Autodesk Inventor part; units mm, degrees
ref_plane "YZ Plane" through (0, 0, 0) normal (1, 0, 0) x (0, 1, 0)
ref_plane "XZ Plane" through (0, 0, 0) normal (0, 1, 0) x (-1, 0, 0)
ref_plane "XY Plane" through (0, 0, 0) normal (0, 0, 1) x (1, 0, 0)
sketch "草图1" plane through (0, 0, 0) normal (0, 0, 1) x (1, 0, 0)
  arc A0 (25, -75) -> (-25, -75) centre (0, -75) ccw
  line L0 (-25, -75) -> (-25, -96.8246)
  line L1 (25, -75) -> (25, -96.8246)
  line L2 (0, 0) -> (9.4022, 0)
  line L3 (0, 0) -> (0, -9.3611)
  arc A1 (75, 25) -> (75, -25) centre (75, 0) ccw
  line L4 (75, -25) -> (96.8246, -25)
  line L5 (75, 25) -> (96.8246, 25)
  arc A2 (-25, 75) -> (25, 75) centre (0, 75) ccw
  line L6 (25, 75) -> (25, 96.8246)
  line L7 (-25, 75) -> (-25, 96.8246)
  arc A3 (-75, -25) -> (-75, 25) centre (-75, 0) ccw
  line L8 (-75, 25) -> (-96.8246, 25)
  line L9 (-75, -25) -> (-96.8246, -25)
  arc A4 (-25, 96.8246) -> (-96.8246, 25) centre (0, 0) ccw
  arc A5 (96.8246, 25) -> (25, 96.8246) centre (0, 0) ccw
  arc A6 (-96.8246, -25) -> (-25, -96.8246) centre (0, 0) ccw
  arc A7 (25, -96.8246) -> (96.8246, -25) centre (0, 0) ccw
  dimension "d0" = 50
  dimension "d2" = 9.4022
  dimension "d3" = 9.3611
  dimension "d6" = 360
  dimension "d12" = 100
extrude "拉伸1" add sketch "草图1" along normal blind 28
sketch "草图2" plane through (0, 0, 28) normal (0, 0, 1) x (1, 0, 0)
  circle A0 centre (0, 0) radius 25
  arc A1 (30, -75) -> (-30, -75) centre (0, -75) ccw
  arc A2 (25, -75) -> (-25, -75) centre (0, -75) ccw
  line L0 (30, -75) -> (30, -90.1388)
  line L1 (-30, -75) -> (-30, -90.1388)
  arc A3 (75, 30) -> (75, -30) centre (75, 0) ccw
  line L2 (75, 30) -> (90.1388, 30)
  line L3 (75, -30) -> (90.1388, -30)
  arc A4 (-30, 75) -> (30, 75) centre (0, 75) ccw
  line L4 (-30, 75) -> (-30, 90.1388)
  line L5 (30, 75) -> (30, 90.1388)
  arc A5 (-75, -30) -> (-75, 30) centre (-75, 0) ccw
  line L6 (-75, -30) -> (-90.1388, -30)
  line L7 (-75, 30) -> (-90.1388, 30)
  arc A6 (-90.1388, -30) -> (-30, -90.1388) centre (0, 0) ccw
  arc A7 (-30, 90.1388) -> (-90.1388, 30) centre (0, 0) ccw
  arc A8 (30, -90.1388) -> (90.1388, -30) centre (0, 0) ccw
  arc A9 (90.1388, 30) -> (30, 90.1388) centre (0, 0) ccw
  dimension "d15" = 50
  dimension "d17" = 5
  dimension "d20" = 360
  dimension "d22" = 95
extrude "拉伸2" cut sketch "草图2" against normal blind 9
pattern_linear "矩形阵列1" count 2 spacing 19 along (0, 0, -1) of "拉伸2"
sketch "草图3" plane through (0, 0, 28) normal (0, 0, 1) x (1, 0, 0)
  circle A0 centre (0, 0) radius 15
  line L0 (-4, 14.4568) -> (4, 14.4568)
  line L1 (4, 14.4568) -> (4, 17.2)
  line L2 (4, 17.2) -> (-4, 17.2)
  line L3 (-4, 17.2) -> (-4, 14.4568)
  dimension "d28" = 30
  dimension "d29" = 17.2
  dimension "d30" = 8
extrude "拉伸3" cut sketch "草图3" against normal blind 28
properties part number "基准图-装填桶"
Geometry: final body of the model. Coordinates: model frame, mm. A direction names the side the tool comes from. Round coordinates to 2 decimals unless told otherwise and drop trailing zeros. Loops run counter-clockwise (first coordinate to the right, second up) from the corner with the lowest first, then second, coordinate; pieces in that order, holes last. Notation, with made-up numbers: M 79,35 L 116,35 A18 cw 116,46 Z; hole C 53,10.25 d6. An arc over 180 degrees is marked long. Put each result on its own line as item: value. Start each with the question number.
(1) Section query A-A (y = 0). Return loops of the section in (x, z).
(2) Draft query along Y for faces 1 (the face through (70.18, 71.24, 13.8)), 2 (the face through (66.74, -67.61, 4.56)), 3 (the face through (-0.5, -49.8, 0)). Return one class per face: +Y half, -Y half, draft (parallel to the pull), parting line (faces both ways), or undercut.
(3) Section query D-D (x = 40.5). Return loops of the section in (y, z), then the cut area to 3 significant figures.
(4) Section query C-C (z = 2.5). State how many separate pieces and enclosed holes the cut face has, then the cut area to 3 significant figures.
(5) Set-up query: faces 4 (the face through (25, -86, 14)), 5 (the face through (25, 86, 14)), 6 (the face through (-86, 25, 14)), 7 (the face through (-82, -30, 24)), 8 (the face through (45.007, 0.66, 4.563)). Return all of +Z, -Z, +X, -X, +Y, -Y with unobstructed straight access to the full face (end or side cutting, diameter ignored); none if empty.
(6) Section query B-B (x = -70). Return loops of the section in (y, z), then the cut area to 3 significant figures.
(7) Contact query for flat-ended pins moving along their axis: pin 1 Ø7 at (x, z) = (82.5, 25.5) entering from +Y; pin 2 Ø7 at (x, z) = (-82.5, 22.5) entering from -Y; pin 3 Ø6.5 at (x, z) = (89, 9) entering from -Y. Output: stop coordinate, or through.
(8) Material intervals for line 1 along X through (y, z) = (0, 16.75); line 2 along X through (y, z) = (-85.5, 26.75); line 3 along Y through (x, z) = (-5.5, 2.5), sorted ascending. Write a range as [from, to].
Findings below:
1. outline: M -50,0 L -45,0 L -45,9 L -25,9 L -25,0 L -15,0 L -15,28 L -25,28 L -25,19 L -45,19 L -45,28 L -50,28 Z; M 15,0 L 25,0 L 25,9 L 45,9 L 45,0 L 50,0 L 50,28 L 45,28 L 45,19 L 25,19 L 25,28 L 15,28 Z
2. face 1: +Y half
2. face 2: undercut
2. face 3: draft
3. outline: M -91.43,0 L -85.93,0 L -85.93,9 L 85.93,9 L 85.93,0 L 91.43,0 L 91.43,28 L 85.93,28 L 85.93,19 L -85.93,19 L -85.93,28 L -91.43,28 Z
3. area: 2,030 mm2
4. separate pieces: 2
4. enclosed holes: 2
4. area: 5,650 mm2
5. face 4: +Z, -Z, -Y
5. face 5: +Z, -Z, +Y
5. face 6: +Z, -Z, -X
5. face 7: +Z
5. face 8: -Z
6. outline: M -71.41,0 L -64.23,0 L -64.23,9 L -29.58,9 L -29.58,0 L -24.49,0 L -24.49,28 L -29.58,28 L -29.58,19 L -64.23,19 L -64.23,28 L -71.41,28 Z; M 24.49,0 L 29.58,0 L 29.58,9 L 64.23,9 L 64.23,0 L 71.41,0 L 71.41,28 L 64.23,28 L 64.23,19 L 29.58,19 L 29.58,28 L 24.49,28 Z
6. area: 1,380 mm2
7. pin 1: stops at y = 61.31
7. pin 2: stops at y = -61.31
7. pin 3: stops at y = -51.45
8. line 1: x = [-50, -15], [15, 50]
8. line 2: x = [-51.86, -41.41], [-30, -25], [25, 30], [41.41, 51.86]
8. line 3: y = [-50.61, -45.51], [-24.39, -13.96], [13.96, 24.39], [45.51, 50.61]
